from build123d import *

# Parameters (mm, degrees)
BOSS_EXTRUDE3_DEPTH   = 72.39
BOSS_EXTRUDE4_DEPTH   = 51.39
F_3_0MM_DOWEL_HOLE4_D = 3


with BuildPart() as part:
    # Sketch1 → Boss-Extrude3 (new body)
    with BuildSketch(Plane(origin=(0, 0, 0), x_dir=(1, 0, 0), z_dir=(0, 1, 0))):
        with BuildLine():
            Line((-11.1466884, 17.698170271), (-23.8485284, 17.698170271))
            Line((-23.8485284, 17.698170271), (-23.8485284, 14.523170271))
            Line((-23.8485284, 14.523170271), (36.9033116, 14.523170271))
            Line((36.9033116, 14.523170271), (36.9033116, 17.698170271))
            Line((36.9033116, 17.698170271), (24.2033116, 17.698170271))
            Line((24.2033116, 17.698170271), (24.2033116, 31.16592192))
            Line((24.2033116, 31.16592192), (18.979662229, 31.16592192))
            ThreePointArc((18.979662229, 31.16592192), (6.479662229, 18.665921919), (-6.020337771, 31.16592192))
            Line((-6.020337771, 31.16592192), (-11.1466884, 31.16592192))
            Line((-11.1466884, 31.16592192), (-11.1466884, 17.698170271))
        make_face()
    extrude(amount=BOSS_EXTRUDE3_DEPTH)

    # Sketch1<13> → Boss-Extrude4 (add)
    with BuildSketch(Plane(origin=(0, 0, 0), x_dir=(1, 0, 0), z_dir=(0, 1, 0))):
        with BuildLine():
            Line((-6.020337771, 31.16592192), (-5.720337771, 31.16592192))
            ThreePointArc((-5.720337771, 31.16592192), (6.479662229, 18.965921919), (18.679662229, 31.16592192))
            Line((18.679662229, 31.16592192), (18.979662229, 31.16592192))
            ThreePointArc((18.979662229, 31.16592192), (6.479662229, 18.665921919), (-6.020337771, 31.16592192))
        make_face()
    extrude(amount=BOSS_EXTRUDE4_DEPTH)

    # Ø3.0mm Dowel Hole4 (through all)
    with Locations(Plane(origin=(0, 0, -31.16592192), x_dir=(-1, 0, 0), z_dir=(0, 0, -1))):
        with Locations((-22.1133116, 66.04), (9.0566884, 66.04), (8.9066884, 6.35), (-21.9633116, 6.35)):
            Hole(F_3_0MM_DOWEL_HOLE4_D / 2)


solid = part.part
The model under review builds one solid part; all positions refer to its coordinate system, in mm. A direction names the side the tool comes from. Round coordinates to 2 decimals unless told otherwise and drop trailing zeros. Order: outer loops, then holes, each group sorted by start corner. A loop starts at its lowest first (then second) coordinate and runs counter-clockwise, first axis right, second up. Notation, with made-up numbers: (50.25, 75.25) -> (108.25, 75.25) arc R14 cw to (108.25, 91.25) -> close; hole circle Ø2 at (-33, 11.5). An arc over 180 degrees is marked (long way). Write item = value, one per line. Start each with the question number.
Item 1: For line 1 along X through (y, z) = (11.5, -26.5); line 2 along Z through (x, y) = (26.5, 63); line 3 along X through (y, z) = (66.04, -20), list the stretches that pass through material, from the lowest coordinate up.
Item 2: Clearance check with flat-ended pins moving along their axes: pin 1 Ø6.5 at (x, y) = (-15.5, 46) entering from -Z; pin 2 Ø4 at (y, z) = (25, -24.5) entering from +X; pin 3 Ø4 at (y, z) = (46.5, -21.5) entering from -X. State where each tip first meets the part, or that it passes through.
Item 3: Consider section A-A on y = 66.04. Write out the cut boundary in (x, z), plus the area to 3 significant figures.
Item 4: Consider section B-B on z = -23. Write out the cut boundary in (x, y), plus the area to 3 significant figures.
Item 5: Mouldability with a two-part tool opening along X and no side actions: class faces 1 (the face through (20.465, 6.416, -22.728)), 2 (the face through (-17, 36, -17.698)), 3 (the face through (36.903, 36, -16)) as released by +X, released by -X, zero draft, split by the parting line, or undercut.
Item 6: For faces 4 (the face through (24.203, 36, -24)), 5 (the face through (-11.147, 36, -25)), 6 (the face through (6.75, 61.74, -18.67)), 7 (the face through (6, 36, -14.523)), 8 (the face through (-10.405, 6.416, -22.728)), list the 3-axis set-ups (+Z, -Z, +X, -X, +Y, -Y) from which the entire face can be reached by the end or side of a thin tool; tool diameter is ignored.
Item 7: Consider section C-C on y = 17. Write out the cut boundary in (x, z), plus the area to 3 significant figures.
Item 8: Consider section D-D on x = -12. Write out the cut boundary in (y, z), plus the area to 3 significant figures.
Conclusion:
q1.line_1 = -11.15 to -4.79, 17.75 to 24.2
q1.line_2 = -17.7 to -14.52
q1.line_3 = -11.15 to -10.56, -7.56 to 0.86, 12.1 to 20.61, 23.61 to 24.2
q2.pin_1 = -17.7
q2.pin_2 = 24.2
q2.pin_3 = -11.15
q3.outline = (-23.85, -17.7) -> (-11.15, -17.7) -> (-11.15, -31.17) -> (-10.56, -31.17) -> (-10.56, -14.52) -> (-23.85, -14.52) -> close; (-7.56, -31.17) -> (-6.02, -31.17) arc R12.5 cw to (18.98, -31.17) -> (20.61, -31.17) -> (20.61, -14.52) -> (-7.56, -14.52) -> close; (23.61, -31.17) -> (24.2, -31.17) -> (24.2, -17.7) -> (36.9, -17.7) -> (36.9, -14.52) -> (23.61, -14.52) -> close
q3.area = 324 mm2
q4.outline = (-11.15, 0) -> (-2.58, 0) -> (-2.58, 51.39) -> (-2.98, 51.39) -> (-2.98, 72.39) -> (-11.15, 72.39) -> close; (15.54, 0) -> (24.2, 0) -> (24.2, 72.39) -> (15.94, 72.39) -> (15.94, 51.39) -> (15.54, 51.39) -> close; hole circle Ø3 at (-9.06, 66.04); hole circle Ø3 at (-8.91, 6.35); hole circle Ø3 at (21.96, 6.35); hole circle Ø3 at (22.11, 66.04)
q4.area = 1,200 mm2
q5.face_1 = undercut
q5.face_2 = zero draft
q5.face_3 = released by +X
q6.face_4 = -Z, +X, +Y, -Y
q6.face_5 = -Z, -X, +Y, -Y
q6.face_6 = -Z, +Y
q6.face_7 = +Z, +X, -X, +Y, -Y
q6.face_8 = +Z, -Z
q7.outline = (-23.85, -17.7) -> (-11.15, -17.7) -> (-11.15, -31.17) -> (-5.72, -31.17) arc R12.2 cw to (18.68, -31.17) -> (24.2, -31.17) -> (24.2, -17.7) -> (36.9, -17.7) -> (36.9, -14.52) -> (-23.85, -14.52) -> close
q7.area = 435 mm2
q8.outline = (0, -17.7) -> (72.39, -17.7) -> (72.39, -14.52) -> (0, -14.52) -> close
q8.area = 230 mm2
